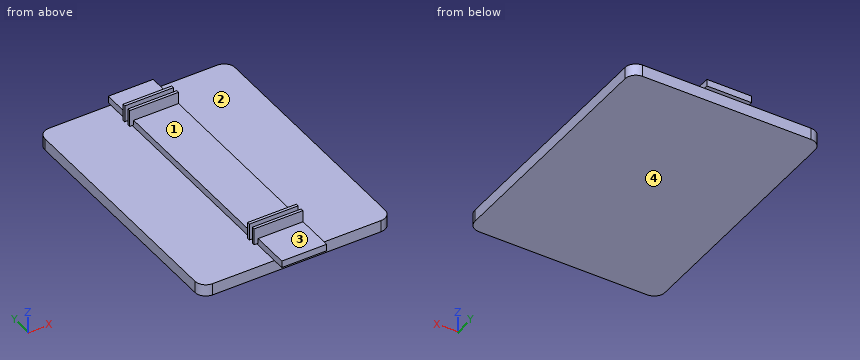
Autodesk Inventor part; units mm, degrees
ref_plane "YZ Plane" through (0, 0, 0) normal (1, 0, 0) x (0, 1, 0)
ref_plane "XZ Plane" through (0, 0, 0) normal (0, 1, 0) x (-1, 0, 0)
ref_plane "XY Plane" through (0, 0, 0) normal (0, 0, 1) x (1, 0, 0)
sketch "Sketch1" plane through (0, 0, 0) normal (0, 0, 1) x (1, 0, 0)
  line L0 (178.3811, -162.3451) -> (-127.8103, -162.3451)
  line L1 (-127.8103, -162.3451) -> (-127.8103, -582.0869)
  line L2 (-127.8103, -582.0869) -> (178.3811, -582.0869)
  line L3 (178.3811, -582.0869) -> (178.3811, -162.3451)
  circle A0 centre (25.2854, -372.216) radius 2.2409
  line L4 (178.3811, -162.3451) -> (-127.8103, -582.0869)
  line L5 (178.3811, -582.0869) -> (-127.8103, -162.3451)
  point P0 (0, 0)
extrude "Extrusion1" add sketch "Sketch1" along normal blind 19.05
sketch "Sketch2" plane through (0, 0, 19.05) normal (0, 0, 1) x (1, 0, 0)
  line L0 (178.3811, -582.0869) -> (-127.8103, -582.0869)
  line L1 (-127.8103, -162.3451) -> (178.3811, -162.3451)
  line L2 (-10.8645, -162.3451) -> (-10.8645, -582.0869)
  circle A0 centre (25.2854, -372.216) radius 4.386
  line L3 (61.4353, -582.0869) -> (61.4353, -162.3451)
  line L4 (-10.8645, -162.3451) -> (61.4353, -582.0869)
  line L5 (61.4353, -162.3451) -> (-10.8645, -582.0869)
  line L6 (-10.8645, -162.3451) -> (61.4353, -162.3451)
  line L7 (61.4353, -582.0869) -> (-10.8645, -582.0869)
  point P0 (0, 0)
  point P1 (25.2854, -372.216)
extrude "Extrusion2" add sketch "Sketch2" along normal blind 11.1125
sketch "Sketch3" plane through (0, 0, 30.1625) normal (0, 0, 1) x (1, 0, 0)
  line L0 (-10.8645, -582.0869) -> (-10.8645, -162.3451)
  line L1 (61.4353, -162.3451) -> (61.4353, -582.0869)
  circle A0 centre (25.2854, -372.216) radius 4.386
  line L2 (-10.8645, -203.9512) -> (61.4353, -203.9512)
  line L3 (61.4353, -203.9512) -> (61.4353, -208.4802)
  line L4 (61.4353, -208.4802) -> (-10.8645, -208.4802)
  line L5 (-10.8645, -208.4802) -> (-10.8645, -203.9512)
  line L6 (-10.8645, -216.6512) -> (61.4353, -216.6512)
  line L7 (61.4353, -216.6512) -> (61.4353, -221.1802)
  line L8 (61.4353, -221.1802) -> (-10.8645, -221.1802)
  line L9 (-10.8645, -221.1802) -> (-10.8645, -216.6512)
  line L10 (25.2854, -372.216) -> (-128.4851, -372.216) construction
  line L11 (-10.8645, -540.4809) -> (61.4353, -540.4809)
  line L12 (61.4353, -540.4809) -> (61.4353, -535.9519)
  line L13 (61.4353, -535.9519) -> (-10.8645, -535.9519)
  line L14 (-10.8645, -535.9519) -> (-10.8645, -540.4809)
  line L15 (61.4353, -527.7809) -> (61.4353, -523.2519)
  line L16 (-10.8645, -523.2519) -> (-10.8645, -527.7809)
  line L17 (-10.8645, -527.7809) -> (61.4353, -527.7809)
  line L18 (61.4353, -523.2519) -> (-10.8645, -523.2519)
  point P0 (0, 0)
  dimension "d6" = 12.7
extrude "Extrusion3" add sketch "Sketch3" along normal blind 19.05 contours L0 L13 L1 L11 | L0 L18 L1 L17 | L0 L6 L1 L8 | L0 L2 L1 L4
fillet "Fillet1" radius 17.4625 4 edges at (-127.8103, -582.0869, 9.525) (-127.8103, -162.3451, 9.525) (178.3811, -582.0869, 9.525) (178.3811, -162.3451, 9.525)
sketch "Sketch4" plane through (-10.8645, -582.0869, 19.05) normal (-1, 0, 0) x (0, 0, 1)
  line L0 (11.1125, 0) -> (11.1125, 41.606)
  line L1 (11.1125, 41.606) -> (30.1625, 41.606)
  line L2 (30.1625, 41.606) -> (30.1625, 46.135)
  line L3 (11.1125, 46.135) -> (30.1625, 46.135)
  line L4 (11.1125, 54.306) -> (30.1625, 54.306)
  line L5 (30.1625, 54.306) -> (30.1625, 58.835)
  line L6 (11.1125, 58.835) -> (30.1625, 58.835)
  line L7 (11.1125, 58.835) -> (11.1125, 360.9067)
  line L8 (11.1125, 360.9067) -> (30.1625, 360.9067)
  line L9 (30.1625, 360.9067) -> (30.1625, 365.4357)
  line L10 (11.1125, 365.4357) -> (30.1625, 365.4357)
  line L11 (11.1125, 373.6067) -> (30.1625, 373.6067)
  line L12 (30.1625, 373.6067) -> (30.1625, 378.1357)
  line L13 (11.1125, 378.1357) -> (30.1625, 378.1357)
  line L14 (0, 0) -> (0, 419.7418)
  line L15 (0, 0) -> (11.1125, 0)
  line L16 (11.1125, 378.1357) -> (3.1565, 378.1357)
  line L17 (3.1565, 378.1357) -> (3.1565, 373.6067)
  line L18 (3.1565, 373.6067) -> (11.1125, 373.6067)
  line L19 (11.1125, 365.4357) -> (3.1565, 365.4357)
  line L20 (3.1565, 365.4357) -> (3.1565, 360.9067)
  line L21 (3.1565, 360.9067) -> (11.1125, 360.9067)
  line L22 (11.1125, 58.835) -> (3.1565, 58.835)
  line L23 (3.1565, 58.835) -> (3.1565, 54.306)
  line L24 (3.1565, 54.306) -> (11.1125, 54.306)
  line L25 (11.1125, 46.135) -> (3.1565, 46.135)
  line L26 (3.1565, 46.135) -> (3.1565, 41.606)
  line L27 (3.1565, 41.606) -> (11.1125, 41.606)
  point P0 (-19.05, 582.0869)
extrude "Extrusion4" add sketch "Sketch4" along normal blind 6.35
sketch "Sketch5" plane through (-10.8645, -582.0869, 30.1625) normal (0, -1, 0) x (1, 0, 0)
  line L0 (0, 0) -> (72.2998, 0)
  line L1 (72.2998, 0) -> (72.2998, -11.1125)
  line L2 (72.2998, -11.1125) -> (0, -11.1125)
  line L3 (0, -11.1125) -> (0, 0)
  point P0 (10.8645, -30.1625)
extrude "Extrusion5" add sketch "Sketch5" along normal blind 19.05
sketch "Sketch6" plane through (-10.8645, -162.3451, 30.1625) normal (0, 1, 0) x (1, 0, 0)
  line L0 (0, 11.1125) -> (72.2998, 11.1125)
  line L1 (72.2998, 11.1125) -> (72.2998, 0)
  line L2 (72.2998, 0) -> (0, 0)
  line L3 (0, 0) -> (0, 11.1125)
  point P0 (10.8645, 30.1625)
extrude "Extrusion6" add sketch "Sketch6" along normal blind 6.35
properties part number "Ruler"
For this review, take the finished solid that the model builds, in its own axes (mm). Face numbers are marked on the shaded views. A direction names the side the tool comes from. Coordinates: 2 decimals unless noted, no trailing zeros. Order: outer loops, then holes, each group sorted by start corner. A loop starts at its lowest first (then second) coordinate and runs counter-clockwise, first axis right, second up. Notation, with made-up numbers: (82.25, 81) -> (127.25, 81) arc R19 ccw to (127.25, 118) -> close; hole circle Ø9 at (-21, 83). An arc over 180 degrees is marked (long way). Return JSON: item names as keys, results as strings.
1. We need section D-D on z = 11.5. Write out the cut boundary in (x, y) (1 decimal).
Answer block:
{"outline": "(-127.8, -564.6) arc R17.5 ccw to (-110.3, -582.1) -> (160.9, -582.1) arc R17.5 ccw to (178.4, -564.6) -> (178.4, -179.8) arc R17.5 ccw to (160.9, -162.3) -> (-110.3, -162.3) arc R17.5 ccw to (-127.8, -179.8) -> close"}
2. Machinability: for the marked faces 3 and 4, which of the approach directions +Z, -Z, +X, -X, +Y, -Y give a long, thin tool a straight path to every point of the face, cutting with its end or side? Answer none if there is none.
Answer block:
{"face 3": "+Z, +X, -X, -Y", "face 4": "-Z, +X, -X, +Y, -Y"}
3. We need section A-A on z = 40. Write out the cut boundary in (x, y).
Answer block:
{"outline": "(-17.21, -540.48) -> (61.44, -540.48) -> (61.44, -535.95) -> (-17.21, -535.95) -> close; (-17.21, -527.78) -> (61.44, -527.78) -> (61.44, -523.25) -> (-17.21, -523.25) -> close; (-17.21, -221.18) -> (61.44, -221.18) -> (61.44, -216.65) -> (-17.21, -216.65) -> close; (-17.21, -208.48) -> (61.44, -208.48) -> (61.44, -203.95) -> (-17.21, -203.95) -> close"}
4. We need section C-C on y = -294.5. Write out the cut boundary in (x, z), and give its area (3 significant figures).
Answer block:
{"outline": "(-127.81, 0) -> (178.38, 0) -> (178.38, 19.05) -> (61.44, 19.05) -> (61.44, 30.16) -> (-10.86, 30.16) -> (-10.86, 19.05) -> (-127.81, 19.05) -> close", "area": "6,640 mm²"}
5. We need section B-B on x = 43.5. Write out the cut boundary in (y, z), and give its area (3 significant figures).
Answer block:
{"outline": "(-601.14, 19.05) -> (-582.09, 19.05) -> (-582.09, 0) -> (-162.35, 0) -> (-162.35, 19.05) -> (-156, 19.05) -> (-156, 30.16) -> (-203.95, 30.16) -> (-203.95, 49.21) -> (-208.48, 49.21) -> (-208.48, 30.16) -> (-216.65, 30.16) -> (-216.65, 49.21) -> (-221.18, 49.21) -> (-221.18, 30.16) -> (-523.25, 30.16) -> (-523.25, 49.21) -> (-527.78, 49.21) -> (-527.78, 30.16) -> (-535.95, 30.16) -> (-535.95, 49.21) -> (-540.48, 49.21) -> (-540.48, 30.16) -> (-601.14, 30.16) -> close", "area": "13,300 mm²"}
6. For pin 1 Ø8 at (x, z) = (23, 40.5) entering from +Y; pin 2 Ø3 at (x, z) = (74, 6.5) entering from +Y; pin 3 Ø24 at (x, y) = (12.5, -178.5) entering from +Z, all flat-tipped, find the tip position at first contact; note any pin that passes through.
Answer block:
{"pin 1": "y = -203.95", "pin 2": "y = -162.35", "pin 3": "z = 30.16"}
7. For line 1 (Z direction, x = 107, y = -509); line 2 (X direction, y = -538.5, z = 33.5); line 3 (Y direction, x = 155, z = 2.5), list the stretches that pass through material, from the lowest coordinate up. Write a range as from..to.
Answer block:
{"line 1": "0..19.05", "line 2": "-17.21..61.44", "line 3": "-582.09..-162.35"}
8. The part is to be moulded in two halves that separate along Y. For the marked faces 1 and 2, say which applies: +Y half, -Y half, draft (parallel to the pull), parting line (faces both ways), or undercut.
Answer block:
{"face 1": "undercut", "face 2": "draft"}
